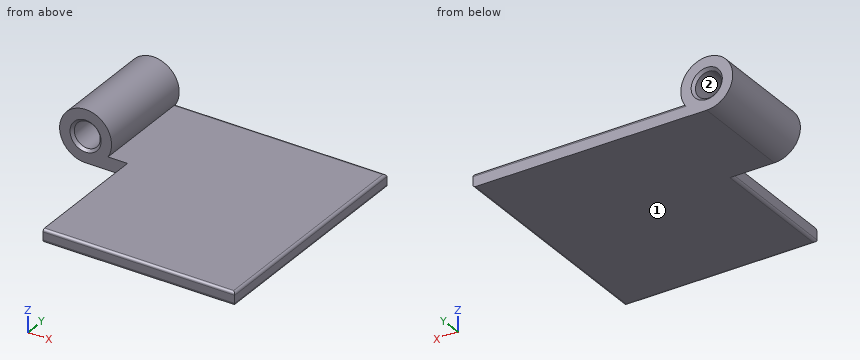
```python
from build123d import *

# Parameters (mm, degrees)
F0_R     = 3.175
F1_DEPTH = 25.4
F0_W     = 46.875538686
F0_H     = 3.175
F2_DEPTH = 57.15
F3_R     = 0.635
F4_SIZE  = 0.635


with BuildPart() as f1:
    # F0 (on Front) → F1 (new body)
    with BuildSketch(Plane.XZ):
        with BuildLine():
            ThreePointArc((5.499261314, -3.175), (-3.175, 5.499261314), (0, -6.35))
            Line((0, -6.35), (10.274461314, -6.35))
            Line((10.274461314, -6.35), (10.274461314, -3.175))
            Line((10.274461314, -3.175), (5.499261314, -3.175))
        make_face()
        Circle(F0_R, mode=Mode.SUBTRACT)
    extrude(amount=F1_DEPTH)

    # F0 (on Front) → F2 (join)
    with BuildSketch(Plane.XZ):
        with Locations((33.712230657, -4.7625)):
            Rectangle(F0_W, F0_H)
    extrude(amount=F2_DEPTH)

    # F3
    f3_edges = [f1.edges().sort_by_distance(p)[0] for p in [
        (33.712231, -57.15, -3.175),
        (33.712231, -57.15, -6.35),
        (57.15, -28.575, -3.175),
        (57.15, -28.575, -6.35),
        (31.324631, 0, -3.175),
        (10.274461, -41.275, -6.35),
    ]]
    fillet(f3_edges, radius=F3_R)

    # F4
    f4_edges = [f1.edges().sort_by_distance(p)[0] for p in [
        (-3.175, -25.4, 0),
        (-3.175, 0, 0),
    ]]
    chamfer(f4_edges, length=F4_SIZE)


solid = f1.part
```
Could you check a few things on this model? Use its own coordinates, in mm. Face numbers are marked on the shaded views. Coordinates: 2 decimals unless noted, no trailing zeros. Loops run counter-clockwise (first coordinate to the right, second up) from the corner with the lowest first, then second, coordinate; pieces in that order, holes last. Notation, with made-up numbers: M 77,15.5 L 102,15.5 A15 cw 102,44.5 Z; hole C 29,49 d9. An arc over 180 degrees is marked long. Put each result on its own line as item: value. Start each with the question number.
(1) Will these pins go through, and if not, where does the flat tip stop? P1, Ø15.5, axis at x = 39, y = -30.5, coming from the +Z side (3 decimals); P2, Ø3, axis at x = 22, z = -2, coming from the +Y side; P3, Ø2, axis at y = -39.5, z = -5, coming from the -X side.
(2) I need wall thicknesses on line 1 (Z direction, x = 0, y = -16.75) (3 decimals); line 2 (Y direction, x = 8.5, z = -5.5); line 3 (Z direction, x = 30.5, y = -36.5) (3 decimals). Which ranges of each line are inside material? Lowest first, please. Write a range as from..to.
(3) Suppose I cut it at A-A on z = 0. Please give me the cut outline in (x, y) (3 decimals).
(4) Suppose I cut it at C-C on x = 30.5. Please give me the cut outline in (y, z) (3 decimals).
(5) Thinking about a two-plate mould opening in X: for the marked faces 1 and 2, which applies, pulls with the +X half, pulls with the -X half, needs draft (parallel to the pull), parting line crosses it, or undercut?
(6) Suppose I cut it at D-D on y = -52. Please give me the cut outline in (x, z) (3 decimals), then the cut area to 3 significant figures.
(7) Suppose I cut it at B-B on y = -11.5. Please give me the cut outline in (x, z) (3 decimals).
Solutions:
1. P1: stops at z = -3.175
1. P2: stops at y = -0.08
1. P3: stops at x = 10.27
2. line 1: z = -6.35..-3.175, 3.175..6.35
2. line 2: y = -25.4..0
2. line 3: z = -6.35..-3.175
3. outline: M -6.35,-25.4 L -3.81,-25.4 L -3.175,-24.765 L -3.175,-0.635 L -3.81,0 L -6.35,0 Z; M 3.175,-24.765 L 3.81,-25.4 L 6.35,-25.4 L 6.35,0 L 3.81,0 L 3.175,-0.635 Z
4. outline: M -57.15,-5.715 A0.635 ccw -56.515,-6.35 L 0,-6.35 L 0,-3.81 A0.635 ccw -0.635,-3.175 L -56.515,-3.175 A0.635 ccw -57.15,-3.81 Z
5. face 1: needs draft
5. face 2: undercut
6. outline: M 10.274,-5.715 A0.635 ccw 10.909,-6.35 L 56.515,-6.35 A0.635 ccw 57.15,-5.715 L 57.15,-3.81 A0.635 ccw 56.515,-3.175 L 10.274,-3.175 Z
6. area: 149 mm2
7. outline: M 0,-6.35 L 56.515,-6.35 A0.635 ccw 57.15,-5.715 L 57.15,-3.81 A0.635 ccw 56.515,-3.175 L 5.499,-3.175 A6.35 ccw long Z; hole C 0,0 d6.35
